Could you check a few things on this model? Use its own coordinates, in mm. Round coordinates to 2 decimals unless told otherwise and drop trailing zeros. Loops run counter-clockwise (first coordinate to the right, second up) from the corner with the lowest first, then second, coordinate; pieces in that order, holes last. Notation, with made-up numbers: (77, 34) -> (127, 34) arc R12 ccw to (127, 46) -> close; hole circle Ø5 at (0.25, -36.75). An arc over 180 degrees is marked (long way). One line per item, written item: value.
```python
from build123d import *

# Parameters (mm, degrees)
F1_DEPTH = 1.27


with BuildPart() as f1:
    # F0 (on Front) → F1 (new body)
    with BuildSketch(Plane.XZ):
        with BuildLine():
            ThreePointArc((3.794874, -0.339167), (3.806217, -0.169752), (3.81, 0))
            Line((3.81, 0), (0, 0))
            Line((0, 0), (3.084668, 0.826534))
            Line((3.084668, 0.826534), (2.998397, 1.148501))
            Line((2.998397, 1.148501), (3.456041, 1.603709))
            ThreePointArc((3.456041, 1.603709), (3.381156, 1.756098), (3.299557, 1.905))
            ThreePointArc((3.299557, 1.905), (3.211897, 2.049345), (3.117927, 2.189664))
            Line((3.117927, 2.189664), (2.493829, 2.022438))
            Line((2.493829, 2.022438), (2.258134, 2.258134))
            Line((2.258134, 2.258134), (2.022438, 2.493829))
            Line((2.022438, 2.493829), (2.191164, 3.116873))
            ThreePointArc((2.191164, 3.116873), (2.050118, 3.211404), (1.905, 3.299557))
            ThreePointArc((1.905, 3.299557), (1.756912, 3.380734), (1.605372, 3.455269))
            Line((1.605372, 3.455269), (1.148501, 2.998397))
            Line((1.148501, 2.998397), (0.826534, 3.084668))
            Line((0.826534, 3.084668), (0.504568, 3.170939))
            Line((0.504568, 3.170939), (0.339167, 3.794874))
            ThreePointArc((0.339167, 3.794874), (0.169752, 3.806217), (0, 3.81))
            ThreePointArc((0, 3.81), (-0.168837, 3.806257), (-0.337341, 3.795036))
            Line((-0.337341, 3.795036), (-0.504568, 3.170939))
            Line((-0.504568, 3.170939), (-0.826534, 3.084668))
            Line((-0.826534, 3.084668), (-1.148501, 2.998397))
            Line((-1.148501, 2.998397), (-1.603709, 3.456041))
            ThreePointArc((-1.603709, 3.456041), (-1.756098, 3.381156), (-1.905, 3.299557))
            ThreePointArc((-1.905, 3.299557), (-2.049345, 3.211897), (-2.189664, 3.117927))
            Line((-2.189664, 3.117927), (-2.022438, 2.493829))
            Line((-2.022438, 2.493829), (-2.258134, 2.258134))
            Line((-2.258134, 2.258134), (-2.493829, 2.022438))
            Line((-2.493829, 2.022438), (-3.116873, 2.191164))
            ThreePointArc((-3.116873, 2.191164), (-3.211404, 2.050118), (-3.299557, 1.905))
            ThreePointArc((-3.299557, 1.905), (-3.380734, 1.756912), (-3.455269, 1.605372))
            Line((-3.455269, 1.605372), (-2.998397, 1.148501))
            Line((-2.998397, 1.148501), (-3.084668, 0.826534))
            Line((-3.084668, 0.826534), (-3.170939, 0.504568))
            Line((-3.170939, 0.504568), (-3.794874, 0.339167))
            ThreePointArc((-3.794874, 0.339167), (-3.806217, 0.169752), (-3.81, 0))
            ThreePointArc((-3.81, 0), (-3.806257, -0.168837), (-3.795036, -0.337341))
            Line((-3.795036, -0.337341), (-3.170939, -0.504568))
            Line((-3.170939, -0.504568), (-3.084668, -0.826534))
            Line((-3.084668, -0.826534), (-2.998397, -1.148501))
            Line((-2.998397, -1.148501), (-3.456041, -1.603709))
            ThreePointArc((-3.456041, -1.603709), (-3.381156, -1.756098), (-3.299557, -1.905))
            ThreePointArc((-3.299557, -1.905), (-3.211897, -2.049345), (-3.117927, -2.189664))
            Line((-3.117927, -2.189664), (-2.493829, -2.022438))
            Line((-2.493829, -2.022438), (-2.258134, -2.258134))
            Line((-2.258134, -2.258134), (-2.022438, -2.493829))
            Line((-2.022438, -2.493829), (-2.191164, -3.116873))
            ThreePointArc((-2.191164, -3.116873), (-2.050118, -3.211404), (-1.905, -3.299557))
            ThreePointArc((-1.905, -3.299557), (-1.756912, -3.380734), (-1.605372, -3.455269))
            Line((-1.605372, -3.455269), (-1.148501, -2.998397))
            Line((-1.148501, -2.998397), (-0.826534, -3.084668))
            Line((-0.826534, -3.084668), (-0.504568, -3.170939))
            Line((-0.504568, -3.170939), (-0.339167, -3.794874))
            ThreePointArc((-0.339167, -3.794874), (-0.169752, -3.806217), (0, -3.81))
            ThreePointArc((0, -3.81), (0.168837, -3.806257), (0.337341, -3.795036))
            Line((0.337341, -3.795036), (0.504568, -3.170939))
            Line((0.504568, -3.170939), (0.826534, -3.084668))
            Line((0.826534, -3.084668), (1.148501, -2.998397))
            Line((1.148501, -2.998397), (1.603709, -3.456041))
            ThreePointArc((1.603709, -3.456041), (1.756098, -3.381156), (1.905, -3.299557))
            ThreePointArc((1.905, -3.299557), (2.049345, -3.211897), (2.189664, -3.117927))
            Line((2.189664, -3.117927), (2.022438, -2.493829))
            Line((2.022438, -2.493829), (2.258134, -2.258134))
            Line((2.258134, -2.258134), (2.493829, -2.022438))
            Line((2.493829, -2.022438), (3.116873, -2.191164))
            ThreePointArc((3.116873, -2.191164), (3.211404, -2.050118), (3.299557, -1.905))
            ThreePointArc((3.299557, -1.905), (3.380734, -1.756912), (3.455269, -1.605372))
            Line((3.455269, -1.605372), (2.998397, -1.148501))
            Line((2.998397, -1.148501), (3.084668, -0.826534))
            Line((3.084668, -0.826534), (3.170939, -0.504568))
            Line((3.170939, -0.504568), (3.794874, -0.339167))
        make_face()
        with BuildLine():
            Line((0, 0), (3.795502, 0.332063))
            ThreePointArc((3.795502, 0.332063), (3.79527, 0.334702), (3.795036, 0.337341))
            Line((3.795036, 0.337341), (3.170939, 0.504568))
            Line((3.170939, 0.504568), (3.084668, 0.826534))
            Line((3.084668, 0.826534), (0, 0))
        make_face()
        with BuildLine():
            Line((0, 0), (3.81, 0))
            ThreePointArc((3.81, 0), (3.806374, 0.16619), (3.795502, 0.332063))
            Line((3.795502, 0.332063), (0, 0))
        make_face()
    extrude(amount=F1_DEPTH)


solid = f1.part
```
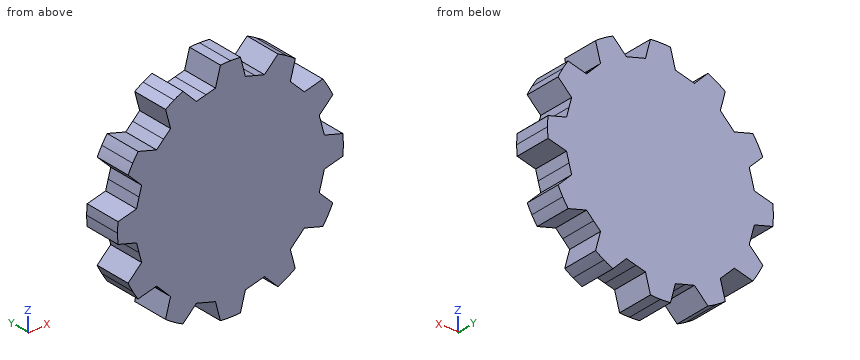
Item 1: If we section it at B-B on x = 1.5: List the corners of the cut face in (y, z) for me, plus the area to 3 significant figures.
Output:
outline: (-1.27, -3.35) -> (0, -3.35) -> (0, 3.35) -> (-1.27, 3.35) -> close
area: 8.51 mm²
Item 2: If we section it at A-A on z = -1.75: List the corners of the cut face in (x, y) for me, plus the area to 3 significant figures.
Output:
outline: (-3.38, -1.27) -> (3.38, -1.27) -> (3.38, 0) -> (-3.38, 0) -> close
area: 8.60 mm²
Item 3: I need wall thicknesses on line 1 (Z direction, x = -3.25, y = -0.15); line 2 (Z direction, x = -1.5, y = -0.95); line 3 (Z direction, x = -1.75, y = -0.1). Which ranges of each line are inside material? Lowest first, please. Write a range as from..to.
Output:
line 1: z = -1.99..-1.4, -0.48..0.48, 1.4..1.99
line 2: z = -3.35..3.35
line 3: z = -3.38..3.38
